Could you check a few things on this model? Use its own coordinates, in mm. Face numbers are marked on the shaded views. A direction names the side the tool comes from. Give positions to 0.01 mm unless a question says otherwise; leave off trailing zeros. Loops run counter-clockwise (first coordinate to the right, second up) from the corner with the lowest first, then second, coordinate; pieces in that order, holes last. Notation, with made-up numbers: (-23.5, 46) -> (22.5, 46) arc R24 ccw to (22.5, 57) -> close; hole circle Ø6 at (-39.5, 52.25). An arc over 180 degrees is marked (long way). Write item = value, one per line. Start each with the question number.
1) I want a section at A-A (z = 0). List the corners of the cut face in (x, y) for me.
2) I need wall thicknesses on probe 1 along Y at (x, z) = (9.75, -1.25); probe 2 along Z at (x, y) = (-0.5, -14). Which ranges of each line are inside material? Lowest first, please. Write a range as from..to.
3) I want a section at D-D (x = -4.5). List the corners of the cut face in (y, z) for me, and give its area (3 significant figures).
4) I want a section at B-B (x = 0). List the corners of the cut face in (y, z) for me.
5) On a 3-axis mill with a long thin cutter (end or side, diameter ignored), from which of +Z, -Z, +X, -X, +Y, -Y can I reach the whole of each face in a straight line? I mean the marked faces 1, 2 and 3. Say none if no direction works.
6) I'm going to push flat-ended pins straight in: pin 1 Ø8 at (y, z) = (2.5, -2.5) entering from +X; pin 2 Ø10 at (x, z) = (-5, 4) entering from -Y; pin 3 Ø3 at (x, z) = (7.5, -4.5) entering from +Y; pin 4 Ø2 at (x, y) = (4.5, -22) entering from +Z. Where does each tip first touch, or does it pass through?
7) I want a section at C-C (y = 2). List the corners of the cut face in (x, z) for me, and give its area (3 significant figures).
from build123d import *

# Parameters (mm, degrees)
CHAMFER1_SIZE = 0.3
CHAMFER2_SIZE = 0.5


with BuildPart() as part:
    # Sketch1 → Revolve1 (revolve)
    with BuildSketch(Plane.XY):
        Polygon((0, -38.6), (2.5, -38.6), (2.5, -31.6), (10.5, -31.6), (10.5, -10.5), (2.5, -10.5), (2.5, 22.2), (0, 22.2), align=None)
    revolve(axis=Axis((0, 22.2, 0), (0, -1, 0)))

    # Chamfer1
    chamfer1_edges = [part.edges().sort_by_distance(p)[0] for p in [
        (-2.5, -38.6, 0),
    ]]
    chamfer(chamfer1_edges, length=CHAMFER1_SIZE)

    # Chamfer2
    chamfer2_edges = [part.edges().sort_by_distance(p)[0] for p in [
        (-2.5, 22.2, 0),
    ]]
    chamfer(chamfer2_edges, length=CHAMFER2_SIZE)


solid = part.part
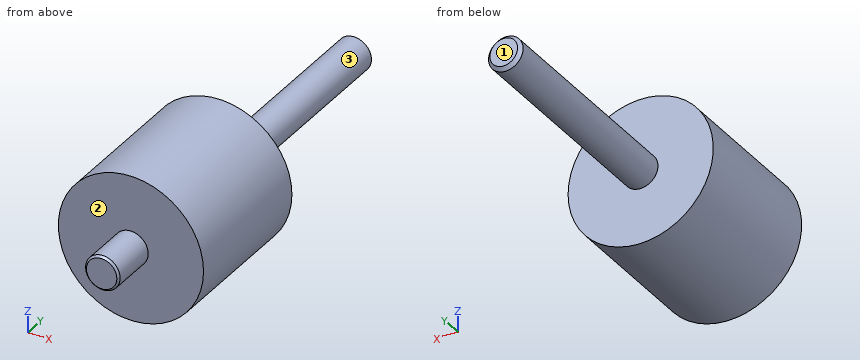
Answer list:
q1.outline = (-10.5, -31.6) -> (-2.5, -31.6) -> (-2.5, -38.3) -> (-2.2, -38.6) -> (2.2, -38.6) -> (2.5, -38.3) -> (2.5, -31.6) -> (10.5, -31.6) -> (10.5, -10.5) -> (2.5, -10.5) -> (2.5, 21.7) -> (2, 22.2) -> (-2, 22.2) -> (-2.5, 21.7) -> (-2.5, -10.5) -> (-10.5, -10.5) -> close
q2.probe_1 = -31.6..-10.5
q2.probe_2 = -10.49..10.49
q3.outline = (-31.6, -9.49) -> (-10.5, -9.49) -> (-10.5, 9.49) -> (-31.6, 9.49) -> close
q3.area = 400 mm^2
q4.outline = (-38.6, -2.2) -> (-38.3, -2.5) -> (-31.6, -2.5) -> (-31.6, -10.5) -> (-10.5, -10.5) -> (-10.5, -2.5) -> (21.7, -2.5) -> (22.2, -2) -> (22.2, 2) -> (21.7, 2.5) -> (-10.5, 2.5) -> (-10.5, 10.5) -> (-31.6, 10.5) -> (-31.6, 2.5) -> (-38.3, 2.5) -> (-38.6, 2.2) -> close
q5.face_1 = +Z, -Z, +X, -X, +Y
q5.face_2 = -Y
q5.face_3 = +Y
q6.pin_1 = 2.5
q6.pin_2 = -38.6
q6.pin_3 = -10.5
q6.pin_4 = 9.9
q7.outline = circle Ø5 at (0, 0)
q7.area = 19.6 mm^2
